from build123d import *


with BuildPart() as part:
    # Sketch1 → Revolve1 (revolve)
    with BuildSketch(Plane.XY):
        with BuildLine():
            Line((50, 90), (50, 115))
            ThreePointArc((50, 115), (0, 165), (-50, 115))
            Line((-50, 115), (-50, 90))
            Line((-50, 90), (-39.896370289, 72.5))
            Line((-39.896370289, 72.5), (-30.95, 72.5))
            Line((-30.95, 72.5), (-28.063248654, 67.5))
            Line((-28.063248654, 67.5), (-2, 50))
            Line((-2, 50), (-2, 22.5))
            Line((-2, 22.5), (-40, 22.5))
            Line((-40, 22.5), (-40, 10))
            Line((-40, 10), (0, 10))
            Line((0, 10), (25, 10))
            Line((25, 10), (25, 22.5))
            Line((25, 22.5), (2, 22.5))
            Line((2, 22.5), (2, 50))
            Line((2, 50), (28.063248654, 67.5))
            Line((28.063248654, 67.5), (30.95, 72.5))
            Line((30.95, 72.5), (39.896370289, 72.5))
            Line((39.896370289, 72.5), (50, 90))
        make_face()
    revolve(axis=Axis((0, 0, 0), (-1, 0, 0)))


solid = part.part
The model under review builds one solid part; all positions refer to its coordinate system, in mm. A direction names the side the tool comes from. Round coordinates to 2 decimals unless told otherwise and drop trailing zeros. Loops run counter-clockwise (first coordinate to the right, second up) from the corner with the lowest first, then second, coordinate; pieces in that order, holes last. Notation, with made-up numbers: (-6, 44.25) -> (49, 44.25) arc R8 ccw to (49, 53.25) -> close; hole circle Ø9 at (-1.5, -1.5). An arc over 180 degrees is marked (long way). Write item = value, one per line. Start each with the question number.
Item 1: To check wall thickness, follow L1, parallel to Y at x = -4.5, z = -6; L2, parallel to Z at x = -15, y = 0; L3, parallel to Y at x = -38, z = 0. State the ranges of each line that lie inside material, in increasing order.
Item 2: Insertion check: pin 1 (3 mm diameter, centred on x = 24, y = -59.5, fed in from -Z); pin 2 (2 mm diameter, centred on x = -4.5, y = 114.5, fed in from +Z); pin 3 (5 mm diameter, centred on x = 30, y = -84, fed in from -Z). Each pin has a flat end and moves straight along its axis. Give the tip position at first contact, or say it passes through.
Item 3: Mouldability with a two-part tool opening along Y and no side actions: class faces 4 (the conical face through (40.528, -15.954, 71.845)), 5 (the flat face through (-50, -69, 59)) as released by +Y, released by -Y, zero draft, split by the parting line, or undercut.
Item 4: Take a section at B-B on x = -35.5. Give the boundary of the cut face in (y, z), plus the area to 3 significant figures.
Item 5: Take a section at A-A on x = -9. Give the boundary of the cut face in (y, z).
Item 6: For faces 1 (the flat face through (2, -10, 22)), 2 (the flat face through (-2, 10, 22)), 3 (the flat face through (50, 69, 59)), list the 3-axis set-ups (+Z, -Z, +X, -X, +Y, -Y) from which the entire face can be reached by the end or side of a thin tool; tool diameter is ignored.
Result:
q1.L1 = -164.69 to -51.33, -21.69 to -8, 8 to 21.69, 51.33 to 164.69
q1.L2 = -162.7 to -58.73, -22.5 to -10, 10 to 22.5, 58.73 to 162.7
q1.L3 = -147.5 to -72.5, -22.5 to -10, 10 to 22.5, 72.5 to 147.5
q2.pin_1 = -148.34
q2.pin_2 = 119.49
q2.pin_3 = -132.9
q3.face_4 = undercut
q3.face_5 = zero draft
q4.outline = circle Ø300.42 at (0, 0); circle Ø45 at (0, 0); hole circle Ø145 at (0, 0); hole circle Ø20 at (0, 0)
q4.area = 55,600 mm²
q5.outline = circle Ø328.37 at (0, 0); circle Ø45 at (0, 0); hole circle Ø109.4 at (0, 0); hole circle Ø20 at (0, 0)
q6.face_1 = +X
q6.face_2 = -X
q6.face_3 = +Z, -Z, +X, +Y, -Y
